Model file for the job. Use its own axes, mm. Give positions to 0.01 mm unless a question says otherwise; leave off trailing zeros. Loops run counter-clockwise (first coordinate to the right, second up) from the corner with the lowest first, then second, coordinate; pieces in that order, holes last. Notation, with made-up numbers: (-13.5, -11) - (31.5, -11) arc R17 ccw to (31.5, -4) - close; hole circle Ø8 at (84.25, 68). An arc over 180 degrees is marked (long way). Use a Markdown table: item, result.
from build123d import *

# Parameters (mm, degrees)
F0_R     = 6
F0_R_2   = 1.95
F1_DEPTH = 8.5
F2_R     = 1.5
F4_R     = 0.35


# Not quite as in the source:
# - a fillet or chamfer that OpenCascade refuses, or shapes differently, is made with other operations: its cross-section is extruded or revolved along the edge and cut away or added


with BuildPart() as f1:
    # F0 (on Top) → F1 (new body)
    with BuildSketch(Plane.XY):
        Circle(F0_R)
        with Locations((-0.5, 0)):
            Circle(F0_R_2, mode=Mode.SUBTRACT)
    extrude(amount=F1_DEPTH)

    # F2
    f2_edges = [f1.edges().sort_by_distance(p)[0] for p in [
        (-6, 0, 8.5),
    ]]
    fillet(f2_edges, radius=F2_R)

    # F3: chamfer of 3 x 2.6078602134 on 1 edges, made by hand

    # F3_s1 → F3_t2 (revolve, cut)
    with BuildSketch(Plane.XZ):
        Polygon((4.0578602134, 8.5), (1.45, 5.5), (1.45, 8.5), align=None)
    revolve(axis=Axis((-0.5, 0, 8.5), (0, 0, 1)), mode=Mode.SUBTRACT)

    # F4
    f4_edges = [f1.edges().sort_by_distance(p)[0] for p in [
        (2.985849, -2.936486, 8.5),
        (2.985849, 2.936486, 8.5),
        (-4.987173, -4e-06, 8.418683),
    ]]
    fillet(f4_edges, radius=F4_R)


solid = f1.part
(1) Pin check, flat tips, straight feed: P1, Ø1.5, axis at y = -3.5, z = 4, coming from the +X side; P2, Ø3, axis at y = 3, z = 2.5, coming from the -X side; P3, Ø5, axis at x = -0.5, y = 0, coming from the -Z side; P4, Ø2, axis at x = -4, z = 5, coming from the -Y side. Stop position of each tip, or through.
Computed:
| item | result |
|---|---|
| P1 | x = 5.33 |
| P2 | x = -5.81 |
| P3 | z = 0 |
| P4 | y = -5.2 |
(2) Mould opens along X. For faces 1 (the flat face through (1.25, -1.25, 0)), 2 (the conical face through (1.476, 0.622, 5.64)), 3 (the cylindrical face through (-6, 0, 3)) say: pulls with the +X half, pulls with the -X half, needs draft (parallel to the pull), parting line crosses it, or undercut.
Computed:
| item | result |
|---|---|
| face 1 | needs draft |
| face 2 | undercut |
| face 3 | parting line crosses it |
(3) Slice it at B-B, the plane z = 6. Write the cut outline in (x, y), plus the area to 3 significant figures.
Computed:
| item | result |
|---|---|
| outline | circle Ø12 at (0, 0); hole circle Ø4.77 at (-0.5, 0) |
| area | 95.2 mm² |
(4) Slice it at A-A, the plane z = 1.25. Write the cut outline in (x, y).
Computed:
| item | result |
|---|---|
| outline | circle Ø12 at (0, 0); hole circle Ø3.9 at (-0.5, 0) |
(5) Drill centre lines: probe 1 along X at (y, z) = (0.5, 5); probe 2 along Y at (x, z) = (-0.5, 2.25); probe 3 along Y at (x, z) = (-2.25, 8.25). Where is each one in solid material? Low to high. Write a range as [from, to].
Computed:
| item | result |
|---|---|
| probe 1 | [-5.98, -2.38], [1.38, 5.98] |
| probe 2 | [-5.98, -1.95], [1.95, 5.98] |
| probe 3 | [-4.83, -3.97], [3.97, 4.83] |
